Source: CAD feature listing. Evaluate the final solid. Frame: model axes, mm. Face numbers are marked on the shaded views. A direction names the side the tool comes from. Round coordinates to 2 decimals unless told otherwise and drop trailing zeros. Loops run counter-clockwise (first coordinate to the right, second up) from the corner with the lowest first, then second, coordinate; pieces in that order, holes last. Notation, with made-up numbers: (-29, 37.25) -> (-16, 37.25) arc R25 cw to (-16, 56.25) -> close; hole circle Ø4 at (60.5, 37.5). An arc over 180 degrees is marked (long way). Put each result on its own line as item: value. Start each with the question number.
1. Contact query for flat-ended pins moving along their axis: pin 1 (9.5 mm diameter, centred on x = 1, y = 1.5, fed in from -Z); pin 2 (4 mm diameter, centred on x = -12.73, y = -12.73, fed in from -Z); pin 3 (2 mm diameter, centred on x = 12.73, y = 12.73, fed in from -Z); pin 4 (4 mm diameter, centred on y = -2, z = 26, fed in from +X). Output: stop coordinate, or through.
2. Cut plane A-A (y = 0). Return the cut outline in (x, z), then the cut area to 3 significant figures.
3. Cut plane C-C (y = 19). Return the cut outline in (x, z), then the cut area to 3 significant figures.
4. Cut plane B-B (z = -7.5). Return the cut outline in (x, y).
5. Set-up query: the marked faces 1, 2 and 3. Return all of +Z, -Z, +X, -X, +Y, -Y with unobstructed straight access to the full face (end or side cutting, diameter ignored); none if empty.
6. Material intervals for L1, parallel to Y at x = 0, z = 24; L2, parallel to X at y = -7.5, z = -4; L3, parallel to Y at x = -12.5, z = -4, sorted ascending.
7. Cut plane D-D (z = 0). Return the cut outline in (x, y).
8. Draft query along X for the marked faces 4, 5, 6 and 7. Return one class per face: pulls with the +X half, pulls with the -X half, needs draft (parallel to the pull), parting line crosses it, or undercut.
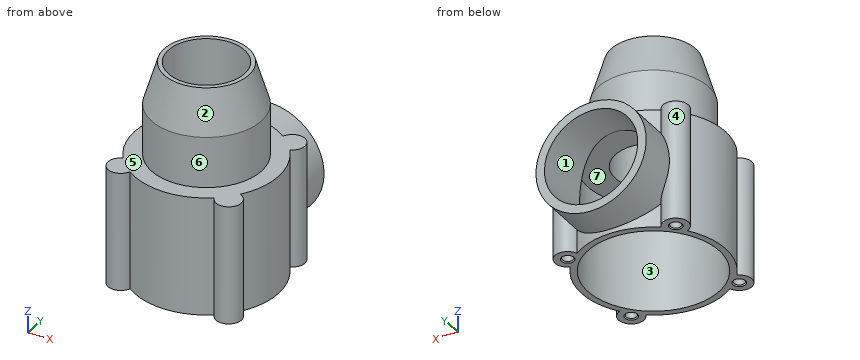
```python
from build123d import *

# Parameters (mm, degrees)
SKETCH1_R           = 17
BOSS_EXTRUDE1_DEPTH = 14
SKETCH2_R           = 13
BOSS_EXTRUDE2_DEPTH = 22
SKETCH3_R           = 13
BOSS_EXTRUDE3_DEPTH = 25
SKETCH4_R           = 15.5
CUT_EXTRUDE1_DEPTH  = 25
SKETCH5_R           = 9
CUT_EXTRUDE2_DEPTH  = 25
CHAMFER2_SIZE       = 10
CHAMFER2_SIZE2      = 3
BOSS_EXTRUDE4_DEPTH = 28
CIRPATTERN1_COUNT   = 4
SKETCH6_R           = 11
CUT_EXTRUDE3_DEPTH  = 25
CIRPATTERN2_COUNT   = 4


with BuildPart() as part:
    # Sketch1 → Boss-Extrude1 (new body, symmetric)
    with BuildSketch(Plane.XY):
        Circle(SKETCH1_R)
    extrude(amount=BOSS_EXTRUDE1_DEPTH, both=True)

    # Sketch2 → Boss-Extrude2 (add)
    with BuildSketch(Plane.XY.offset(14)):
        Circle(SKETCH2_R)
    extrude(amount=BOSS_EXTRUDE2_DEPTH)

    # Sketch3 → Boss-Extrude3 (add)
    with BuildSketch(Plane(origin=(0, 0, 0), x_dir=(1, 0, 0), z_dir=(0, 1, 0))):
        with Locations(Location((0, 0, 0), (0, 0, 90))):  # turned: the seam where the file's is
            Circle(SKETCH3_R)
    extrude(amount=BOSS_EXTRUDE3_DEPTH)

    # Sketch4 → Cut-Extrude1 (cut)
    with BuildSketch(Plane(origin=(0, 0, -14), x_dir=(-1, 0, 0), z_dir=(0, 0, -1))):
        Circle(SKETCH4_R)
    extrude(amount=-CUT_EXTRUDE1_DEPTH, mode=Mode.SUBTRACT)

    # Sketch5 → Cut-Extrude2 (cut)
    with BuildSketch(Plane.XY.offset(36)):
        Circle(SKETCH5_R)
    extrude(amount=-CUT_EXTRUDE2_DEPTH, mode=Mode.SUBTRACT)

    # Chamfer2
    chamfer2_edges = [part.edges().sort_by_distance(p)[0] for p in [
        (-13, 0, 36),
    ]]
    chamfer2_side = [part.faces().sort_by_distance(p)[0] for p in [
        (-13, 0, 25),
    ]]
    chamfer(chamfer2_edges, length=CHAMFER2_SIZE, length2=CHAMFER2_SIZE2, reference=chamfer2_side[0])

    # Sketch7 → Boss-Extrude4 (add)
    with BuildSketch(Plane(origin=(0, 0, -14), x_dir=(-1, 0, 0), z_dir=(0, 0, -1))):
        with BuildLine():
            ThreePointArc((-9.819351092, 11.992928922), (-14.849242405, 14.849242405), (-11.992928922, 9.819351092))
            ThreePointArc((-11.992928922, 9.819351092), (-10.960155108, 10.960155108), (-9.819351092, 11.992928922))
        make_face()
    boss_extrude4 = extrude(amount=-BOSS_EXTRUDE4_DEPTH)

    # CirPattern1: Boss-Extrude4 ×4 about axis
    cirpattern1_axis = Axis((0, 0, 0), (0, 0, 1))
    for i in range(1, CIRPATTERN1_COUNT):
        add(boss_extrude4.rotate(cirpattern1_axis, i * 360 / CIRPATTERN1_COUNT))

    # Sketch6 → Cut-Extrude3 (cut)
    with BuildSketch(Plane(origin=(0, 25, 0), x_dir=(1, 0, 0), z_dir=(0, 1, 0))):
        with Locations(Location((0, 0, 0), (0, 0, 270))):  # turned: the seam where the file's is
            Circle(SKETCH6_R)
    extrude(amount=-CUT_EXTRUDE3_DEPTH, mode=Mode.SUBTRACT)

    # Sketch9 → Tap Drill for M3x0.5 Tap1 (revolve, cut)
    with BuildSketch(Plane(origin=(12.727922061, 12.727922061, -14), x_dir=(0, 1, 0), z_dir=(1, 0, 0))):
        Polygon((0, 0), (0, 9.751075774), (1.25, 9), (1.25, 0.25), (1.5, 0), align=None)
    tap_drill_for_m3x0_5_tap1 = revolve(axis=Axis((12.727922061, 12.727922061, -20.35), (0, 0, 1)), mode=Mode.SUBTRACT)

    # CirPattern2: Tap Drill for M3x0.5 Tap1 ×4 about axis
    cirpattern2_axis = Axis((0, 0, 0), (0, 0, 1))
    for i in range(1, CIRPATTERN2_COUNT):
        add(tap_drill_for_m3x0_5_tap1.rotate(cirpattern2_axis, i * 360 / CIRPATTERN2_COUNT), mode=Mode.SUBTRACT)


solid = part.part
```
Solution:
1. pin 1: passes through
1. pin 2: stops at z = -14
1. pin 3: stops at z = -4.85
1. pin 4: stops at x = 13
2. outline: (-17, -14) -> (-15.5, -14) -> (-15.5, 11) -> (-9, 11) -> (-9, 36) -> (-10, 36) -> (-13, 26) -> (-13, 14) -> (-17, 14) -> close; (9, 11) -> (15.5, 11) -> (15.5, -14) -> (17, -14) -> (17, 14) -> (13, 14) -> (13, 26) -> (10, 36) -> (9, 36) -> close
2. area: 269 mm^2
3. outline: circle Ø26 at (0, 0); hole circle Ø22 at (0, 0)
3. area: 151 mm^2
4. outline: (-13.8, -9.93) arc R3 ccw (long way) to (-9.93, -13.8) arc R17 ccw to (9.93, -13.8) arc R3 ccw (long way) to (13.8, -9.93) arc R17 ccw to (13.8, 9.93) arc R3 ccw (long way) to (10.62, 14.86) -> (10.62, 25) -> (8.05, 25) -> (8.05, 13.25) arc R15.5 cw (long way) to (-8.05, 13.25) -> (-8.05, 25) -> (-10.62, 25) -> (-10.62, 14.86) arc R3 ccw (long way) to (-13.8, 9.93) arc R17 ccw to start; hole circle Ø2.5 at (-12.73, -12.73); hole circle Ø2.5 at (-12.73, 12.73); hole circle Ø2.5 at (12.73, -12.73); hole circle Ø2.5 at (12.73, 12.73)
5. face 1: +Y
5. face 2: +Z
5. face 3: -Z
6. L1: y = -13 to -9, 9 to 13
6. L2: x = -15.26 to -13.56, 13.56 to 15.26
6. L3: y = -15.72 to -9.17, 9.17 to 15.72
7. outline: (-13.8, -9.93) arc R3 ccw (long way) to (-9.93, -13.8) arc R17 ccw to (9.93, -13.8) arc R3 ccw (long way) to (13.8, -9.93) arc R17 ccw to (13.8, 9.93) arc R3 ccw to (13, 15.72) -> (13, 25) -> (11, 25) -> (11, 10.92) arc R15.5 cw (long way) to (-11, 10.92) -> (-11, 25) -> (-13, 25) -> (-13, 15.72) arc R3 ccw to (-13.8, 9.93) arc R17 ccw to start
8. face 4: undercut
8. face 5: needs draft
8. face 6: parting line crosses it
8. face 7: undercut
